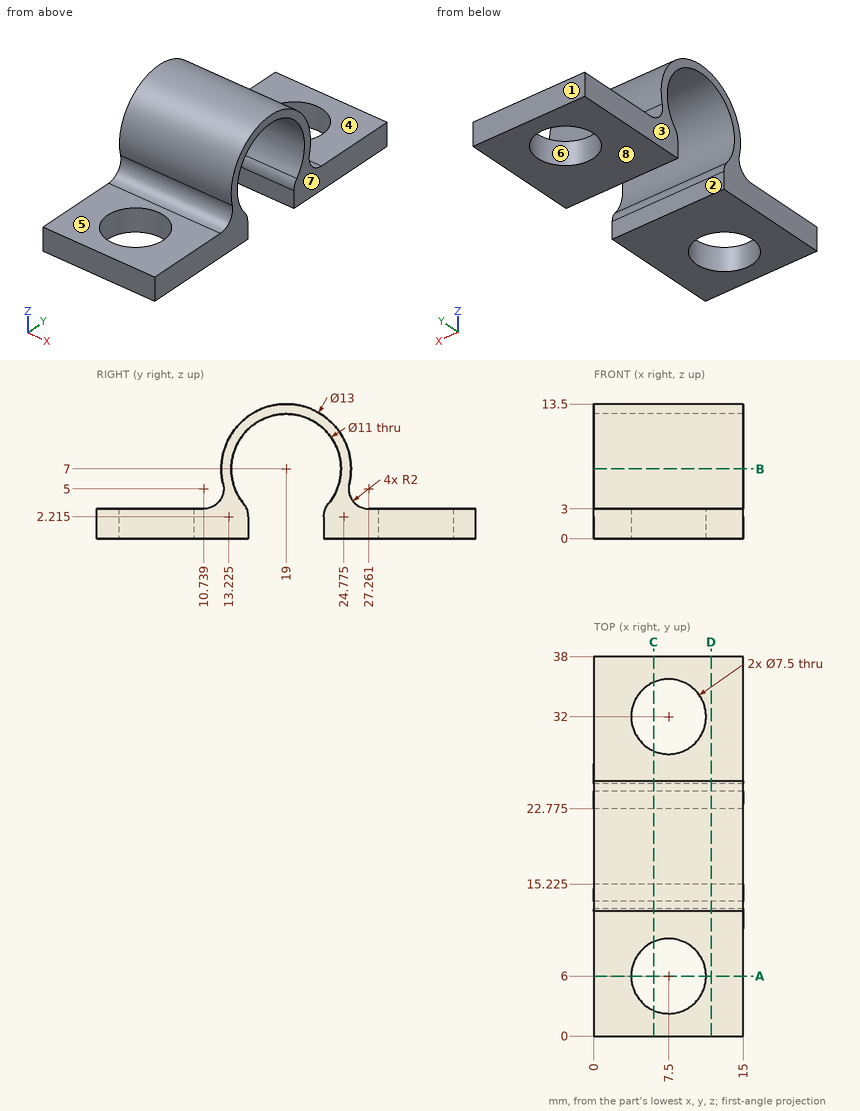
Study the drawing (mm; zero at the part's minimum x, y, z) and answer. A direction names the side the tool comes from. Give positions to 0.01 mm unless a question says otherwise; leave off trailing zeros. Order: outer loops, then holes, each group sorted by start corner. A loop starts at its lowest first (then second) coordinate and runs counter-clockwise, first axis right, second up. Notation, with made-up numbers: M 51,28 L 67,28 A21 cw 67,61 Z; hole C 22.5,-13 d3. An arc over 180 degrees is marked long. Put each result on its own line as item: value. Start each with the question number.
Item 1: The part is cut by section D-D, the plane x = 11.75. Determine the outline of the cut face in (y, z) (1 decimal), and give its area (3 significant figures).
Item 2: Flat-ended cylindrical pins translate along their axes: P1, Ø6, axis at x = 3.5, z = 8, coming from the +Y side; P2, Ø8.5, axis at x = 5, y = 8, coming from the +Z side; P3, Ø2.5, axis at x = 9.5, z = 1.5, coming from the -Y side; P4, Ø8.5, axis at x = 11, y = 32.5, coming from the +Z side. Find the tip coordinate at first contact, or state that the pin passes through.
Item 3: The part is cut by section C-C, the plane x = 6. Determine the outline of the cut face in (y, z) (1 decimal).
Item 4: For a pull along X with two mould halves and no side action, classify the marked faces 6, 7 and 8 as +X half, -X half, draft (parallel to the pull), parting line (faces both ways), or undercut.
Item 5: Find the intervals of material crossed by line 1 along Y through (x, z) = (5.25, 7); line 2 along Z through (x, y) = (11.5, 36.5); line 3 along Y through (x, z) = (13.25, 3.5) (1 decimal), in increasing order.
Item 6: Which of the six approach directions +Z, -Z, +X, -X, +Y, -Y give full straight-line access (tool end or side, diameter ignored) to the marked faces 1, 2, 3, 4 and 5?
Item 7: The part is cut by section A-A, the plane y = 6. Determine the outline of the cut face in (x, z), and give its area (3 significant figures).
Item 8: The part is cut by section B-B, the plane z = 7. Determine the outline of the cut face in (x, y).
Answer key:
1. outline: M 0,0 L 15.2,0 L 15.2,2.2 A2 ccw 14.8,3.5 A5.5 cw long 23.2,3.5 A2 ccw 22.8,2.2 L 22.8,0 L 38,0 L 38,3 L 27.3,3 A2 cw 25.3,5.5 A6.5 ccw long 12.7,5.5 A2 cw 10.7,3 L 0,3 Z
1. area: 123 mm²
2. P1: stops at y = 25.5
2. P2: stops at z = 3.69
2. P3: stops at y = 0
2. P4: stops at z = 3
3. outline: M 0,0 L 2.6,0 L 2.6,3 L 0,3 Z; M 9.4,0 L 15.2,0 L 15.2,2.2 A2 ccw 14.8,3.5 A5.5 cw long 23.2,3.5 A2 ccw 22.8,2.2 L 22.8,0 L 28.6,0 L 28.6,3 L 27.3,3 A2 cw 25.3,5.5 A6.5 ccw long 12.7,5.5 A2 cw 10.7,3 L 9.4,3 Z; M 35.4,0 L 38,0 L 38,3 L 35.4,3 Z
4. face 6: undercut
4. face 7: +X half
4. face 8: draft
5. line 1: y = 12.5 to 13.5, 24.5 to 25.5
5. line 2: z = 0 to 3
5. line 3: y = 12.1 to 14.8, 23.2 to 25.9
6. face 1: +Z, -Z, +X, -X, +Y
6. face 2: -Z, +X, -X
6. face 3: +Z, -Z, -X, +Y, -Y
6. face 4: +Z, +X, -X, +Y
6. face 5: +Z, +X, -X, -Y
7. outline: M 0,0 L 3.75,0 L 3.75,3 L 0,3 Z; M 11.25,0 L 15,0 L 15,3 L 11.25,3 Z
7. area: 22.5 mm²
8. outline: M 0,12.5 L 15,12.5 L 15,13.5 L 0,13.5 Z; M 0,24.5 L 15,24.5 L 15,25.5 L 0,25.5 Z
